```python
from build123d import *
from OCP.BRepFilletAPI import BRepFilletAPI_MakeFillet

# Parameters (mm, degrees)
SKETCH1_R           = 32.5
BOSS_EXTRUDE1_DEPTH = 10
FILLET1_R1          = 5
FILLET1_R2          = 2
BOSS_EXTRUDE2_DEPTH = 30
CIRPATTERN1_COUNT   = 4


with BuildPart() as part:
    # Sketch1 → Boss-Extrude1 (new body)
    with BuildSketch(Plane(origin=(0, 0, 0), x_dir=(1, 0, 0), z_dir=(0, 1, 0))):
        with Locations(Location((0, 0, 0), (0, 0, 270))):
            Circle(SKETCH1_R)
    boss_extrude1 = extrude(amount=-BOSS_EXTRUDE1_DEPTH)

    # Sketch2 → Revolve1 (revolve)
    with BuildSketch(Plane(origin=(0, 0, 0), x_dir=(0, 0, -1), z_dir=(1, 0, 0))):
        Polygon((0, 0), (0, 22), (22, 22), (22, 18), (25, 13), (25, 0), align=None)
    revolve(axis=Axis((0, 0, 0), (0, 1, 0)))

    # Fillet1: one fillet with a radius per group of edges: ONE call of the kernel's fillet builder (fillet() takes one radius for all edges)
    fillet1_edges_1 = [part.edges().sort_by_distance(p)[0] for p in [
        (0, 18, 22),
        (0, 13, 25),
    ]]
    fillet1_edges_2 = [part.edges().sort_by_distance(p)[0] for p in [
        (0, 22, 22),
    ]]
    fillet1 = BRepFilletAPI_MakeFillet(part.part.solid().wrapped)
    for e in fillet1_edges_1:
        fillet1.Add(FILLET1_R1, e.wrapped)
    for e in fillet1_edges_2:
        fillet1.Add(FILLET1_R2, e.wrapped)
    add(Compound.cast(fillet1.Shape()), mode=Mode.REPLACE)

    # Sketch3 → Boss-Extrude2 (add)
    with BuildSketch(Plane(origin=(0, 0, 0), x_dir=(0, 0, -1), z_dir=(1, 0, 0))):
        with BuildLine():
            Line((1.25, 11.615080175), (-1.25, 11.615080175))
            Line((-1.25, 11.615080175), (-1.25, 5.615080175))
            ThreePointArc((-1.25, 5.615080175), (0, 4.544871187), (1.25, 5.615080175))
            Line((1.25, 5.615080175), (1.25, 11.615080175))
        make_face()
    boss_extrude2 = extrude(amount=BOSS_EXTRUDE2_DEPTH)

    # CirPattern1: Boss-Extrude1, Boss-Extrude2 ×4 about axis
    cirpattern1_axis = Axis((0, 0, 0), (0, 1, 0))
    add([boss_extrude1.rotate(cirpattern1_axis, i * 360 / CIRPATTERN1_COUNT) for i in range(1, CIRPATTERN1_COUNT)])
    add([boss_extrude2.rotate(cirpattern1_axis, i * 360 / CIRPATTERN1_COUNT) for i in range(1, CIRPATTERN1_COUNT)])


solid = part.part
```
Geometry check sheet. Reference: the model listing, model coordinates, mm. A direction names the side the tool comes from. Give positions to 0.01 mm unless a question says otherwise; leave off trailing zeros. Write each loop counter-clockwise with the first axis right and the second up, starting at its lowest first coordinate (ties: lowest second). Pieces come first, ordered by that corner, then holes.
1) Material ranges on L1, parallel to Y at x = -18, z = 17.5; L2, parallel to X at y = 2, z = -1; L3, parallel to Y at x = 25.5, z = 1, recorded low to high.
2) Gauge pin test, flat ends, axial feed: pin 1 (1.3 mm diameter, centred on x = 0, z = 27.5, fed in from +Y); pin 2 (2.5 mm diameter, centred on x = -28, y = 9.5, fed in from +Z); pin 3 (1.5 mm diameter, centred on y = 9.5, z = 26.5, fed in from -X). Record the tip position at first contact, or that the pin passes through.
3) Section check A-A, the plane x = 27. Record the boundary of the cut face in (y, z).
4) Section check B-B, the plane y = 3. Record the boundary of the cut face in (x, z), and give its area (3 significant figures).
5) Access from +Z, -Z, +X, -X, +Y, -Y to the whole of each face (thin tool, end or side, straight path). Record for faces 1 (the flat face through (-1.25, 9, 27)), 2 (the flat face through (-30, 8, 0)), 3 (the flat face through (27, 11.615, 0)), 4 (the flat face through (-27, 9, -1.25)), 5 (the cylindrical face through (-0.025, 4.545, 27.449)).
Computed:
1. L1: y = -10 to 0
1. L2: x = -24.98 to 24.98
1. L3: y = -10 to 0, 5.04 to 11.62
2. pin 1: stops at y = 11.62
2. pin 2: stops at z = 1.25
2. pin 3: stops at x = -1.25
3. outline: (-10, -18.09) - (0, -18.09) - (0, 18.09) - (-10, 18.09) - close; (5.62, -1.25) - (11.62, -1.25) - (11.62, 1.25) - (5.62, 1.25) arc R1.27 ccw to start
4. outline: circle Ø50 at (0, 0)
4. area: 1,960 mm2
5. face 1: +Z, -X, +Y
5. face 2: +Z, -Z, -X, +Y
5. face 3: +Z, -Z, +X, +Y
5. face 4: -Z, -X, +Y
5. face 5: +Z
